The figure shows three views and two pictorial views of one solid part (mm, origin at its lowest corner). Answer the questions. Coordinates: 2 decimals unless noted, no trailing zeros. Loops run counter-clockwise (first coordinate to the right, second up) from the corner with the lowest first, then second, coordinate; pieces in that order, holes last. Notation, with made-up numbers: (49.25, 39) -> (71.25, 39) arc R7 ccw to (71.25, 44) -> close; hole circle Ø2 at (47, 73.25). An arc over 180 degrees is marked (long way). Answer as a JSON object with one key per item and string values. Group by question number.
1) Flat-ended cylindrical pins translate along their axes: P1, Ø1, axis at y = 1.5, z = 29.5, coming from the -X side; P2, Ø1.6, axis at x = 16, y = 1.5, coming from the +Z side. Find the tip coordinate at first contact, or state that the pin passes through.
2) Section A-A, the plane y = 2.5 is taken. Give the vertices of the cut face in (x, z), plus the area to 3 significant figures.
3) Section B-B, the plane x = 25 is taken. Give the vertices of the cut face in (y, z), plus the area to 3 significant figures.
4) Consider probe 1 along Z at (x, y) = (2, 0.55). Determine where the line is inside the solid, lowest interval first. Write a range as [from, to].
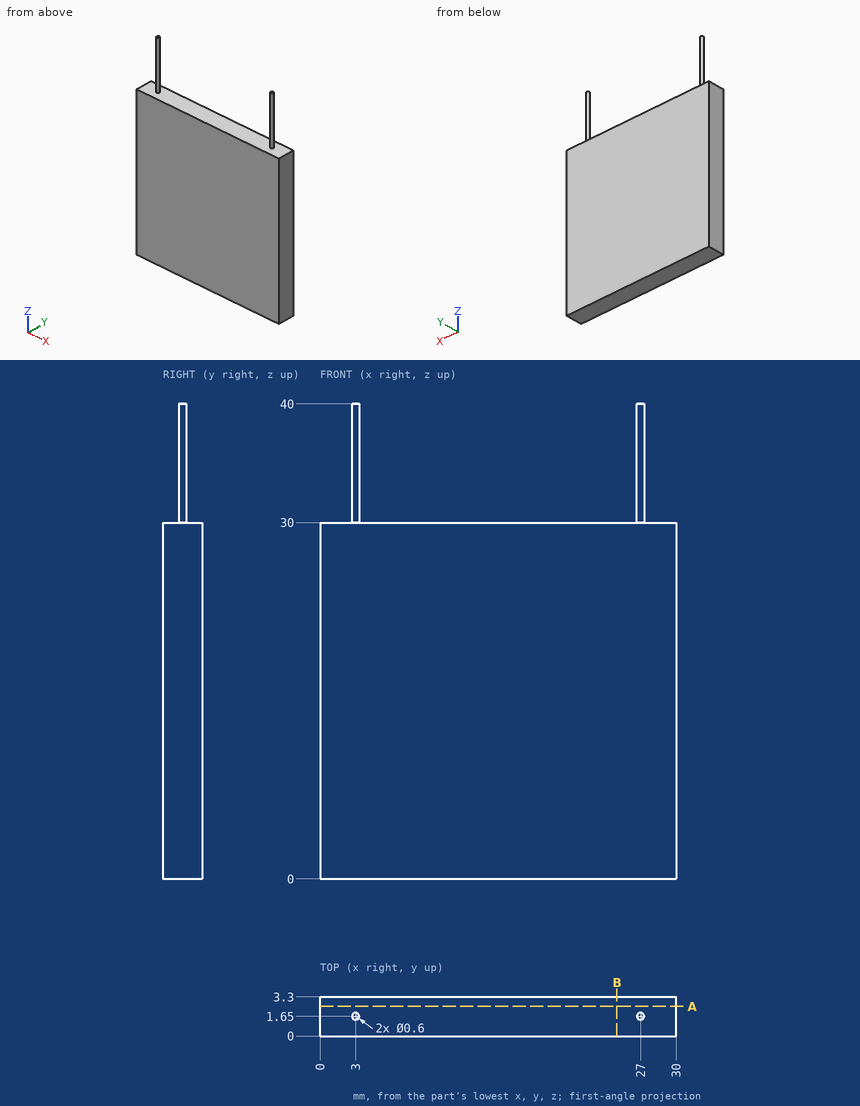
Determined:
{
 "1": {"P1": "x = 0", "P2": "z = 30"},
 "2": {"outline": "(0, 0) -> (30, 0) -> (30, 30) -> (0, 30) -> close", "area": "900 mm²"},
 "3": {"outline": "(0, 0) -> (3.3, 0) -> (3.3, 30) -> (0, 30) -> close", "area": "99.0 mm²"},
 "4": {"probe 1": "[0, 30]"}
}
